Here's how the part is built. I have some questions about the finished solid (model axes, mm). Round coordinates to 2 decimals unless told otherwise and drop trailing zeros. Loops run counter-clockwise (first coordinate to the right, second up) from the corner with the lowest first, then second, coordinate; pieces in that order, holes last. Notation, with made-up numbers: (6, 15) - (17, 15) arc R25 ccw to (17, 51) - close; hole circle Ø8 at (-19.75, 70.25). An arc over 180 degrees is marked (long way). Answer as a JSON object with one key per item and string values. Group by question number.
1) If we mould it in two halves opening along X, with no side actions, what happens to faces 1 (the face through (-2.5, 2, 7)), 2 (the face through (22, 0, 7)), 3 (the face through (20.02, 2.07, 7.4)), 4 (the face through (25.02, 2.07, 7.4))? For each: pulls with the +X half, pulls with the -X half, needs draft (parallel to the pull), parting line crosses it, or undercut.
2) Will this pin go through, and if not, where does the flat tip stop? P1, Ø2, axis at x = 9, y = 2.5, coming from the -Z side.
3) If I drill on line 1 along X through (y, z) = (0.4, 4); line 2 along Y through (x, z) = (1, 10); line 3 along Y through (x, z) = (24.5, 2), over which ranges is the centre line in solid material (lowest first)? Write a range as [from, to].
4) I want a section at A-A, the plane x = 34.5. Please give me the cut outline in (y, z).
Autodesk Inventor part; units mm, degrees
ref_plane "YZ Plane" through (0, 0, 0) normal (1, 0, 0) x (0, 1, 0)
ref_plane "XZ Plane" through (0, 0, 0) normal (0, 1, 0) x (-1, 0, 0)
ref_plane "XY Plane" through (0, 0, 0) normal (0, 0, 1) x (1, 0, 0)
sketch "スケッチ1" plane through (0, 0, 0) normal (0, 0, 1) x (1, 0, 0)
  line L0 (-2.5, 0) -> (47.5, 0)
  arc A0 (-1.2061, 2.7902) -> (1.2061, 2.7902) centre (0, 3.44) ccw
  arc A1 (-1.4749, 3.5744) -> (-1.2061, 2.7902) centre (1.03, 3.995) ccw
  arc A2 (1.2061, 2.7902) -> (1.4749, 3.5744) centre (-1.03, 3.995) ccw
  arc A3 (-1.4749, 3.5744) -> (-1.9779, 4) centre (-1.9779, 3.49) ccw
  arc A4 (1.9779, 4) -> (1.4749, 3.5744) centre (1.9779, 3.49) ccw
  line L1 (1.9779, 4) -> (2.5, 4)
  line L2 (-1.9779, 4) -> (-2.5, 4)
  line L3 (6.9779, 4) -> (7.5, 4)
  arc A5 (6.9779, 4) -> (6.4749, 3.5744) centre (6.9779, 3.49) ccw
  arc A6 (6.2061, 2.7902) -> (6.4749, 3.5744) centre (3.97, 3.995) ccw
  arc A7 (3.7939, 2.7902) -> (6.2061, 2.7902) centre (5, 3.44) ccw
  arc A8 (3.5251, 3.5744) -> (3.7939, 2.7902) centre (6.03, 3.995) ccw
  arc A9 (3.5251, 3.5744) -> (3.0221, 4) centre (3.0221, 3.49) ccw
  line L4 (3.0221, 4) -> (2.5, 4)
  line L5 (11.9779, 4) -> (12.5, 4)
  arc A10 (11.9779, 4) -> (11.4749, 3.5744) centre (11.9779, 3.49) ccw
  arc A11 (11.2061, 2.7902) -> (11.4749, 3.5744) centre (8.97, 3.995) ccw
  arc A12 (8.7939, 2.7902) -> (11.2061, 2.7902) centre (10, 3.44) ccw
  arc A13 (8.5251, 3.5744) -> (8.7939, 2.7902) centre (11.03, 3.995) ccw
  arc A14 (8.5251, 3.5744) -> (8.0221, 4) centre (8.0221, 3.49) ccw
  line L6 (8.0221, 4) -> (7.5, 4)
  line L7 (16.9779, 4) -> (17.5, 4)
  arc A15 (16.9779, 4) -> (16.4749, 3.5744) centre (16.9779, 3.49) ccw
  arc A16 (16.2061, 2.7902) -> (16.4749, 3.5744) centre (13.97, 3.995) ccw
  arc A17 (13.7939, 2.7902) -> (16.2061, 2.7902) centre (15, 3.44) ccw
  arc A18 (13.5251, 3.5744) -> (13.7939, 2.7902) centre (16.03, 3.995) ccw
  arc A19 (13.5251, 3.5744) -> (13.0221, 4) centre (13.0221, 3.49) ccw
  line L8 (13.0221, 4) -> (12.5, 4)
  line L9 (21.9779, 4) -> (22.5, 4)
  arc A20 (21.9779, 4) -> (21.4749, 3.5744) centre (21.9779, 3.49) ccw
  arc A21 (21.2061, 2.7902) -> (21.4749, 3.5744) centre (18.97, 3.995) ccw
  arc A22 (18.7939, 2.7902) -> (21.2061, 2.7902) centre (20, 3.44) ccw
  arc A23 (18.5251, 3.5744) -> (18.7939, 2.7902) centre (21.03, 3.995) ccw
  arc A24 (18.5251, 3.5744) -> (18.0221, 4) centre (18.0221, 3.49) ccw
  line L10 (18.0221, 4) -> (17.5, 4)
  line L11 (26.9779, 4) -> (27.5, 4)
  arc A25 (26.9779, 4) -> (26.4749, 3.5744) centre (26.9779, 3.49) ccw
  arc A26 (26.2061, 2.7902) -> (26.4749, 3.5744) centre (23.97, 3.995) ccw
  arc A27 (23.7939, 2.7902) -> (26.2061, 2.7902) centre (25, 3.44) ccw
  arc A28 (23.5251, 3.5744) -> (23.7939, 2.7902) centre (26.03, 3.995) ccw
  arc A29 (23.5251, 3.5744) -> (23.0221, 4) centre (23.0221, 3.49) ccw
  line L12 (23.0221, 4) -> (22.5, 4)
  line L13 (31.9779, 4) -> (32.5, 4)
  arc A30 (31.9779, 4) -> (31.4749, 3.5744) centre (31.9779, 3.49) ccw
  arc A31 (31.2061, 2.7902) -> (31.4749, 3.5744) centre (28.97, 3.995) ccw
  arc A32 (28.7939, 2.7902) -> (31.2061, 2.7902) centre (30, 3.44) ccw
  arc A33 (28.5251, 3.5744) -> (28.7939, 2.7902) centre (31.03, 3.995) ccw
  arc A34 (28.5251, 3.5744) -> (28.0221, 4) centre (28.0221, 3.49) ccw
  line L14 (28.0221, 4) -> (27.5, 4)
  line L15 (36.9779, 4) -> (37.5, 4)
  arc A35 (36.9779, 4) -> (36.4749, 3.5744) centre (36.9779, 3.49) ccw
  arc A36 (36.2061, 2.7902) -> (36.4749, 3.5744) centre (33.97, 3.995) ccw
  arc A37 (33.7939, 2.7902) -> (36.2061, 2.7902) centre (35, 3.44) ccw
  arc A38 (33.5251, 3.5744) -> (33.7939, 2.7902) centre (36.03, 3.995) ccw
  arc A39 (33.5251, 3.5744) -> (33.0221, 4) centre (33.0221, 3.49) ccw
  line L16 (33.0221, 4) -> (32.5, 4)
  line L17 (41.9779, 4) -> (42.5, 4)
  arc A40 (41.9779, 4) -> (41.4749, 3.5744) centre (41.9779, 3.49) ccw
  arc A41 (41.2061, 2.7902) -> (41.4749, 3.5744) centre (38.97, 3.995) ccw
  arc A42 (38.7939, 2.7902) -> (41.2061, 2.7902) centre (40, 3.44) ccw
  arc A43 (38.5251, 3.5744) -> (38.7939, 2.7902) centre (41.03, 3.995) ccw
  arc A44 (38.5251, 3.5744) -> (38.0221, 4) centre (38.0221, 3.49) ccw
  line L18 (38.0221, 4) -> (37.5, 4)
  line L19 (46.9779, 4) -> (47.5, 4)
  arc A45 (46.9779, 4) -> (46.4749, 3.5744) centre (46.9779, 3.49) ccw
  arc A46 (46.2061, 2.7902) -> (46.4749, 3.5744) centre (43.97, 3.995) ccw
  arc A47 (43.7939, 2.7902) -> (46.2061, 2.7902) centre (45, 3.44) ccw
  arc A48 (43.5251, 3.5744) -> (43.7939, 2.7902) centre (46.03, 3.995) ccw
  arc A49 (43.5251, 3.5744) -> (43.0221, 4) centre (43.0221, 3.49) ccw
  line L20 (43.0221, 4) -> (42.5, 4)
  line L21 (-2.5, 4) -> (-2.5, 0)
  line L22 (47.5, 4) -> (47.5, 0)
  point P0 (0, 0)
  point P1 (0, 2.07)
  point P2 (5, 2.07)
  point P3 (10, 2.07)
  point P4 (15, 2.07)
  point P5 (20, 2.07)
  point P6 (25, 2.07)
  point P7 (30, 2.07)
  point P8 (35, 2.07)
  point P9 (40, 2.07)
  point P10 (45, 2.07)
  dimension "d0" = 1.37
  dimension "d1" = 2.54
  dimension "d2" = 2.54
  dimension "d3" = 1.03
  dimension "d4" = 1.03
  dimension "d5" = 0.51
  dimension "d6" = 0.51
  dimension "d7" = 1.93
  dimension "d9" = 5
  dimension "d10" = 2.5
  dimension "d11" = 4
  dimension "d14" = 5
extrude "押し出し1" add sketch "スケッチ1" along normal blind 15
fillet "フィレット1" radius 0.5 4 edges at (47.5, 0, 7.5) (-2.5, 0, 7.5) (-2.5, 4, 7.5) (47.5, 4, 7.5)
properties part number "belttunagi"
Outcome:
{
 "1": {"face 1": "pulls with the -X half", "face 2": "needs draft", "face 3": "undercut", "face 4": "undercut"},
 "2": {"P1": "z = 0"},
 "3": {"line 1": "[-2.49, 47.49]", "line 2": "[0, 2.5]", "line 3": "[0, 2.16]"},
 "4": {"outline": "(0, 0) - (2.16, 0) - (2.16, 15) - (0, 15) - close"}
}
